Autodesk Fusion 360 part; units mm, degrees
sketch "Sketch1" plane through (0, 0, 0) normal (0, 1, 0) x (1, 0, 0)
  circle A0 centre (0, 0) radius 18 construction
  circle A1 centre (0, 0) radius 14
  circle A2 centre (-16.6298, 6.8883) radius 2.25
  circle A3 centre (-16.6298, -6.8883) radius 2.25
  circle A4 centre (-6.8883, -16.6298) radius 2.25
  circle A5 centre (6.8883, -16.6298) radius 2.25
  circle A6 centre (16.6298, -6.8883) radius 2.25
  circle A7 centre (16.6298, 6.8883) radius 2.25
  circle A8 centre (6.8883, 16.6298) radius 2.25
  circle A9 centre (-6.8883, 16.6298) radius 2.25
  line L0 (-18.5, 7.663) -> (-18.5, -7.663)
  line L1 (-18.5, -7.663) -> (-7.663, -18.5)
  line L2 (-7.663, -18.5) -> (7.663, -18.5)
  line L3 (7.663, -18.5) -> (18.5, -7.663)
  line L4 (18.5, -7.663) -> (18.5, 7.663)
  line L5 (18.5, 7.663) -> (7.663, 18.5)
  line L6 (7.663, 18.5) -> (-7.663, 18.5)
  line L7 (-7.663, 18.5) -> (-18.5, 7.663)
  line L8 (-18.5, 1) -> (18.5, 1)
  point P0 (-16.6298, 6.8883)
  dimension "d1" = 36
  dimension "d2" = 28
  dimension "d3" = 4.5
  dimension "d5" = 360
  dimension "d6" = 18.5
  dimension "d7" = 1
extrude "Extrude1" add sketch "Sketch1" along normal blind 1 contours A1 A2 A7 A8 A9 L0 L4 L5 L6 L7 L8
fillet "Fillet1" radius 0.5 8 edges at (18.5, 0.5, -5.6373) (17.0677, 0.5, -9.0953) (9.0953, 0.5, -17.0677) (5.6373, 0.5, -18.5) (-5.6373, 0.5, -18.5) (-9.0953, 0.5, -17.0677) (-17.0677, 0.5, -9.0953) (-18.5, 0.5, -5.6373)
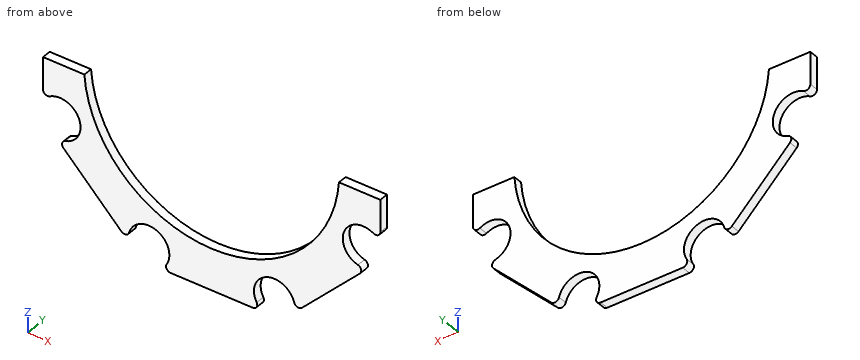
Geometry: final body of the model. Coordinates: model frame, mm. Give positions to 0.01 mm unless a question says otherwise; leave off trailing zeros. Write each loop counter-clockwise with the first axis right and the second up, starting at its lowest first coordinate (ties: lowest second). Pieces come first, ordered by that corner, then holes.
1. Section query B-B, the plane x = -15. Return loops of the section in (y, z), then the cut area to 3 significant figures.
2. Pin query (flat end, axial travel): P1, Ø5, axis at x = -6.89, z = -16.63, coming from the -Y side. Return the tip coordinate at first contact, or that it passes through.
3. Section query D-D, the plane x = 8. Return loops of the section in (y, z).
4. Section query C-C, the plane z = -15. Return loops of the section in (x, y).
5. Line query: probe 1 along X at (y, z) = (0.5, -15.5); probe 2 along X at (y, z) = (0.15, -8.5); probe 3 along X at (y, z) = (0.6, -3.5). Output: solid intervals per line, ascending.
6. Section query A-A, the plane z = -11. Return loops of the section in (x, y).
Computed:
1. outline: (0, -11.16) - (1, -11.16) - (1, -8.44) - (0, -8.44) - close; (0, -5.34) - (1, -5.34) - (1, -1) - (0, -1) - close
1. area: 7.06 mm2
2. P1: stops at y = 0
3. outline: (0, -14.67) - (1, -14.67) - (1, -11.49) - (0, -11.49) - close
4. outline: (-11.16, 0) - (-8.44, 0) - (-8.44, 1) - (-11.16, 1) - close; (-5.34, 0) - (5.34, 0) - (5.34, 1) - (-5.34, 1) - close; (8.44, 0) - (11.16, 0) - (11.16, 1) - (8.44, 1) - close
5. probe 1: x = -10.66 to -8.83, -4.94 to 4.94, 8.83 to 10.66
5. probe 2: x = -15.06 to -11.12, 11.12 to 15.06
5. probe 3: x = -18.5 to -13.56, 13.56 to 18.5
6. outline: (-15.16, 0) - (-8.66, 0) - (-8.66, 1) - (-15.16, 1) - close; (8.66, 0) - (15.16, 0) - (15.16, 1) - (8.66, 1) - close
